For this review, take the finished solid that the model builds, in its own axes (mm). A direction names the side the tool comes from. Coordinates: 2 decimals unless noted, no trailing zeros. Order: outer loops, then holes, each group sorted by start corner. A loop starts at its lowest first (then second) coordinate and runs counter-clockwise, first axis right, second up.
from build123d import *

# Parameters (mm, degrees)
EXTRUDE_1_DEPTH     = 100
SKETCH_5_W          = 100
SKETCH_5_H          = 2
EXTRUDE_1_2_DEPTH   = 45
SKETCH_6_W          = 100
SKETCH_6_H          = 56
CUT_EXTRUDE_1_DEPTH = 124.020020532
SKETCH_7_R          = 4
SKETCH_7_R_2        = 3
EXTRUDE_2_DEPTH     = 3


with BuildPart() as part:
    # 草图1 → Extrude 1 (new body)
    with BuildSketch(Plane.XY):
        Polygon((-48.242261061, 18.127395065), (-48.242261061, -28.872604935), (55.757738939, -28.872604935), (55.757738939, 18.127395065), (53.757738939, 18.127395065), (53.757738939, -26.872604935), (-46.242261061, -26.872604935), (-46.242261061, 18.127395065), align=None)
    extrude(amount=-EXTRUDE_1_DEPTH)

    # 草图5 → Extrude 1 2 (add)
    with BuildSketch(Plane(origin=(0, -26.872604935, 0), x_dir=(1, 0, 0), z_dir=(0, 1, 0))):
        with Locations((3.757738939, 99)):
            Rectangle(SKETCH_5_W, SKETCH_5_H)
    extrude(amount=EXTRUDE_1_2_DEPTH)

    # 草图6 → 切除-拉伸1 (cut, through all)
    with BuildSketch(Plane(origin=(0, -26.872604935, 0), x_dir=(1, 0, 0), z_dir=(0, 1, 0))):
        with Locations((3.757738939, 28)):
            Rectangle(SKETCH_6_W, SKETCH_6_H)
    extrude(amount=-CUT_EXTRUDE_1_DEPTH, mode=Mode.SUBTRACT)

    # 草图7 → 拉伸-薄壁2 (add)
    with BuildSketch(Plane(origin=(-46.242261061, 0, 0), x_dir=(0, 0, -1), z_dir=(1, 0, 0))):
        with Locations((25, -3.872604935)):
            Circle(SKETCH_7_R)
        with Locations((25, -3.872604935)):
            Circle(SKETCH_7_R_2, mode=Mode.SUBTRACT)
    extrude_2 = extrude(amount=EXTRUDE_2_DEPTH)

    # 镜向1: 拉伸-薄壁2 across plane
    add(extrude_2.mirror(Plane(origin=(3.757738939, 0, 0), x_dir=(0, 0, 1), z_dir=(1, 0, 0))))


solid = part.part
1. To check wall thickness, follow L1, parallel to X at y = -8.5, z = -64; L2, parallel to Y at x = -45.45, z = -25; L3, parallel to Y at x = 49.5, z = -74.5. State the ranges of each line that lie inside material, in increasing order.
Answer below:
L1: x = -48.24 to -46.24, 53.76 to 55.76
L2: y = -7.87 to -6.87, -0.87 to 0.13
L3: y = -28.87 to -26.87
2. Take a section at A-A, the plane z = -32. Give the boundary of the cut face in (x, y).
Answer below:
outline: (-48.24, -28.87) - (-46.24, -28.87) - (-46.24, 18.13) - (-48.24, 18.13) - close; (53.76, -28.87) - (55.76, -28.87) - (55.76, 18.13) - (53.76, 18.13) - close
3. Take a section at B-B, the plane y = 14.5. Give the boundary of the cut face in (x, z), plus the area to 3 significant figures.
Answer below:
outline: (-48.24, -100) - (55.76, -100) - (55.76, 0) - (53.76, 0) - (53.76, -98) - (-46.24, -98) - (-46.24, 0) - (-48.24, 0) - close
area: 600 mm2
4. The part is to be moulded in two halves that separate along Z. For faces 5 (the face through (3, -28.873, -83)), 6 (the face through (3, -6, -100)), 7 (the face through (-44.763, -6.534, -26.384)), say which applies: +Z half, -Z half, draft (parallel to the pull), parting line (faces both ways), or undercut.
Answer below:
face 5: draft
face 6: -Z half
face 7: undercut
5. Take a section at C-C, the plane x = 40. Give the boundary of the cut face in (y, z).
Answer below:
outline: (-28.87, -100) - (18.13, -100) - (18.13, -98) - (-26.87, -98) - (-26.87, -56) - (-28.87, -56) - close
6. Clearance check with flat-ended pins moving along their axes: pin 1 Ø1 at (x, y) = (33, -10) entering from +Z; pin 2 Ø1 at (x, y) = (11, -28) entering from +Z. State where each tip first meets the part, or that it passes through.
Answer below:
pin 1: stops at z = -98
pin 2: stops at z = -56
7. Machinability: for faces 1 (the face through (52.279, -6.534, -26.384)), 2 (the face through (-43.242, -2, -22)), 3 (the face through (4, -26.873, -77)), 4 (the face through (-19.6, 18.127, -98.4)), which of the approach directions +Z, -Z, +X, -X, +Y, -Y give a long, thin tool a straight path to every point of the face, cutting with its end or side? Answer none if there is none.
Answer below:
face 1: none
face 2: +Z, +Y, -Y
face 3: +Z, +Y
face 4: +Z, -Z, +X, -X, +Y
